```python
from build123d import *

# Parameters (mm, degrees)
F0_W     = 50
F0_H     = 50
F0_R     = 2
F0_R_2   = 2.1
F1_DEPTH = 3
F2_D     = 4.5


# Not quite as in the source:
# - a feature names something its author has since deleted; it is built from what else it names


with BuildPart() as f1:
    # F0 (on Top) → F1 (new body)
    with BuildSketch(Plane.XY):
        with Locations((-3.725e-07, 2.55218e-05)):
            Rectangle(F0_W, F0_H)
        with Locations((-17.5000003725, -17.4999744782)):
            Circle(F0_R, mode=Mode.SUBTRACT)
        with Locations((17.4999996275, -17.4999744782)):
            Circle(F0_R, mode=Mode.SUBTRACT)
        Circle(F0_R_2, mode=Mode.SUBTRACT)
        with Locations((-17.5000003725, 17.5000255218)):
            Circle(F0_R, mode=Mode.SUBTRACT)
        with Locations((17.4999996275, 17.5000255218)):
            Circle(F0_R, mode=Mode.SUBTRACT)
    extrude(amount=F1_DEPTH)

    # F2 (through all)
    with Locations(Plane(origin=(0, 0, 0), x_dir=(1, 0, 0), z_dir=(0, 0, -1))):
        with Locations((-17.5000003725, 17.4999744782), (-17.5000003725, -17.5000255218), (17.4999996275, -17.5000255218), (17.4999996275, 17.4999744782)):
            Hole(F2_D / 2)


solid = f1.part
```
The model under review builds one solid part; all positions refer to its coordinate system, in mm. Coordinates: 2 decimals unless noted, no trailing zeros. Order: outer loops, then holes, each group sorted by start corner. A loop starts at its lowest first (then second) coordinate and runs counter-clockwise, first axis right, second up. Notation, with made-up numbers: (-21.75, 58.5) -> (22.25, 58.5) arc R17 ccw to (22.25, 63.5) -> close; hole circle Ø11 at (6.25, 51). An arc over 180 degrees is marked (long way). Answer in a Markdown table with one row per item. Add a question column.
Item 1: To check wall thickness, follow probe 1 along Y at (x, z) = (17.5, 1.45); probe 2 along Y at (x, z) = (0, 1.1); probe 3 along X at (y, z) = (-17, 2.7). State the ranges of each line that lie inside material, in increasing order.
Item 2: We need section A-A on x = -17.5. Write out the cut boundary in (y, z).
Item 3: We need section D-D on z = 0.65. Write out the cut boundary in (x, y), plus the area to 3 significant figures.
Item 4: Mouldability with a two-part tool opening along X and no side actions: class faces 1 (the flat face through (-25, 0, 1)), 2 (the cylindrical face through (19.16, 15.98, 1.52)), 3 (the flat face through (0, 25, 1)), 4 (the cylindrical face through (2.003, 0.631, 1.479)) as +X half, -X half, draft (parallel to the pull), parting line (faces both ways), or undercut.
Item 5: Clearance check with a flat-ended pin moving along its axis: pin 1 (4 mm diameter, centred on x = 0, y = 0, fed in from +Z) (3 decimals). State where the tip first meets the part, or that it passes through.
Item 6: We need section B-B on y = 0. Write out the cut boundary in (x, z).
Final values:
| question | item | result |
|---|---|---|
| 1 | probe 1 | y = -25 to -19.75, -15.25 to 15.25, 19.75 to 25 |
| 1 | probe 2 | y = -25 to -2.1, 2.1 to 25 |
| 1 | probe 3 | x = -25 to -19.69, -15.31 to 15.31, 19.69 to 25 |
| 2 | outline | (-25, 0) -> (-19.75, 0) -> (-19.75, 3) -> (-25, 3) -> close; (-15.25, 0) -> (15.25, 0) -> (15.25, 3) -> (-15.25, 3) -> close; (19.75, 0) -> (25, 0) -> (25, 3) -> (19.75, 3) -> close |
| 3 | outline | (-25, -25) -> (25, -25) -> (25, 25) -> (-25, 25) -> close; hole circle Ø4.5 at (-17.5, -17.5); hole circle Ø4.5 at (-17.5, 17.5); hole circle Ø4.2 at (0, 0); hole circle Ø4.5 at (17.5, -17.5); hole circle Ø4.5 at (17.5, 17.5) |
| 3 | area | 2,420 mm2 |
| 4 | face 1 | -X half |
| 4 | face 2 | undercut |
| 4 | face 3 | draft |
| 4 | face 4 | undercut |
| 5 | pin 1 | passes through |
| 6 | outline | (-25, 0) -> (-2.1, 0) -> (-2.1, 3) -> (-25, 3) -> close; (2.1, 0) -> (25, 0) -> (25, 3) -> (2.1, 3) -> close |
